Geometry check sheet. Reference: the model listing, model coordinates, mm. A direction names the side the tool comes from. Coordinates: 2 decimals unless noted, no trailing zeros. Loops run counter-clockwise (first coordinate to the right, second up) from the corner with the lowest first, then second, coordinate; pieces in that order, holes last. Notation, with made-up numbers: (8.25, 9) - (60.25, 9) arc R15 ccw to (60.25, 32) - close; hole circle Ø7 at (-2.5, -38). An arc over 180 degrees is marked (long way). Write each question's results on one line, items separated by ' | '. Start each with the question number.
(1) Material ranges on probe 1 along Z at (x, y) = (-18, -39.5); probe 2 along Y at (x, z) = (-25, 39.5); probe 3 along Z at (x, y) = (38.5, 23), recorded low to high.
(2) Go/stop test with flat-tipped pins: pin 1 Ø2 at (x, z) = (-6.5, 159) entering from -Y; pin 2 Ø4 at (x, y) = (37, 4) entering from +Z; pin 3 Ø6 at (x, y) = (-18, -18.5) entering from +Z. Record where each tip stops, or that it passes through.
(3) Sectioned sample at A-A (z = 115). Enter the section's corners in (x, y).
(4) Access from +Z, -Z, +X, -X, +Y, -Y to the whole of each face (thin tool, end or side, straight path). Record for faces 4 (the face through (-1, 49.437, 50)), 5 (the face through (0, -1.363, 49)).
(5) Mould release check, pull along Z, two halves, no side actions. Record for faces 1 (the face through (-31, -11, 101.6)), 2 (the face through (0.09, -50.25, 99.79)), 3 (the face through (48.36, -50.35, 51.42)): pulls with the +Z half, pulls with the -Z half, needs draft (parallel to the pull), parting line crosses it, or undercut.
from build123d import *

# Parameters (mm, degrees)
F0_W     = 101.6
F0_H     = 101.6
F1_DEPTH = 101.6
F2_R     = 25.4
F3_DEPTH = 25.4
F4_DEPTH = 101.6
F7_W     = 50.8
F7_H     = 50.8
F8_DEPTH = 50.8
F9_R     = 6.35


with BuildPart() as f1:
    # F0 (on Top) → F1 (new body)
    with BuildSketch(Plane.XY):
        with Locations((-0.531297791, -1.3627031267)):
            Rectangle(F0_W, F0_H)
    extrude(amount=F1_DEPTH)

    # F2 (on face) → F3 (join)
    with BuildSketch(Plane.XY.offset(101.6)):
        Circle(F2_R)
    extrude(amount=F3_DEPTH)

    # F4 (add): a face of the model
    f4_faces = [f1.faces().sort_by_distance(p)[0] for p in [
        (0, 0, 127),
    ]]
    extrude(f4_faces, amount=F4_DEPTH)

    # F5 (on face) → F6 (revolve)
    with BuildSketch(Plane.XY.offset(228.6)):
        with BuildLine():
            Line((0, -25.4), (0, -38.1))
            ThreePointArc((0, -38.1), (38.1, 0), (0, 38.1))
            Line((0, 38.1), (0, 25.4))
            ThreePointArc((0, 25.4), (17.9605122421, 17.9605122421), (25.4, 0))
            ThreePointArc((25.4, 0), (17.9605122421, -17.9605122421), (0, -25.4))
        make_face()
        with BuildLine():
            Line((0, 25.4), (0, -25.4))
            ThreePointArc((0, -25.4), (17.9605122421, -17.9605122421), (25.4, 0))
            ThreePointArc((25.4, 0), (17.9605122421, 17.9605122421), (0, 25.4))
        make_face()
    revolve(axis=Axis((0, 0, 228.6), (0, -1, 0)))

    # F7 (on face) → F8 (cut)
    with BuildSketch(Plane.XZ.offset(52.1627031267)):
        with Locations((0, 48.9108748734)):
            Rectangle(F7_W, F7_H)
    extrude(amount=-F8_DEPTH, mode=Mode.SUBTRACT)

    # F9
    f9_edges = [f1.edges().sort_by_distance(p)[0] for p in [
        (50.268702, -1.362703, 101.6),
        (50.268702, -1.362703, 0),
        (50.268702, -52.162703, 50.8),
        (50.268702, 49.437297, 50.8),
        (-0.531298, -52.162703, 101.6),
        (-51.331298, -52.162703, 50.8),
        (-0.531298, -52.162703, 0),
        (-51.331298, -1.362703, 0),
        (-0.531298, 49.437297, 0),
        (-0.531298, 49.437297, 101.6),
        (-51.331298, -1.362703, 101.6),
        (-51.331298, 49.437297, 50.8),
        (-25.4, 0, 200.201937),
        (-25.4, 0, 101.6),
    ]]
    fillet(f9_edges, radius=F9_R)


solid = f1.part
Outcome:
1) probe 1: z = 0 to 23.51, 74.31 to 101.6 | probe 2: y = -1.36 to 49.44 | probe 3: z = 0 to 101.6
2) pin 1: stops at y = -24.8 | pin 2: stops at z = 243.14 | pin 3: stops at z = 259.12
3) outline: circle Ø50.8 at (0, 0)
4) face 4: +Z, -Z, +X, -X, +Y | face 5: -Y
5) face 1: undercut | face 2: pulls with the +Z half | face 3: needs draft
